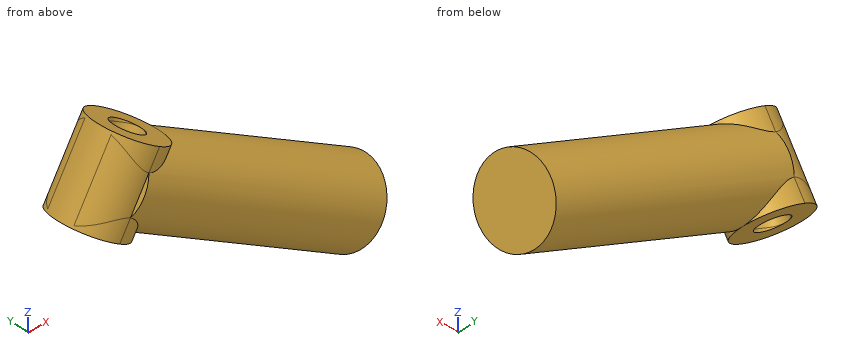
```python
from build123d import *
from build123d.topology import SkipClean

# Parameters (mm, degrees)
BOSS_EXTRUDE1_DEPTH = 25
SKETCH2_R           = 8
CUT_EXTRUDE1_DEPTH  = 110
CUT_EXTRUDE2_DEPTH  = 150
BOSS_EXTRUDE2_START = 21.60254038
BOSS_EXTRUDE2_DEPTH = 21.60254038
SKETCH5_R           = 13
CUT_EXTRUDE3_DEPTH  = 50
SKETCH6_R           = 13
BOSS_EXTRUDE3_DEPTH = 100
SKETCH7_R           = 5
CUT_EXTRUDE4_DEPTH  = 50
SKETCH8_R           = 11.5
SKETCH8_R_2         = 5
BOSS_EXTRUDE4_DEPTH = 13
CUT_EXTRUDE5_DEPTH  = 28


with BuildPart() as part:
    # Sketch1 → Boss-Extrude1 (new, symmetric)
    with BuildSketch(Plane(origin=(0, 0, 0), x_dir=(1, 0, 0), z_dir=(0, 1, 0))):
        Polygon((86.602540378, 150), (103.923048454, 160), (114.724318643, 141.291651246), (93.073683549, 128.791651246), (158.073683549, 16.208348754), (179.724318643, 28.708348754), (190.525588833, 10), (173.205080757, 0), (45.59802172, 0), (22.79901086, 39.489045172), align=None)
    extrude(amount=BOSS_EXTRUDE1_DEPTH, both=True)

    # Sketch2 → Cut-Extrude1 (cut, symmetric)
    with BuildSketch(Plane(origin=(140.729128115, 0, -81.25), x_dir=(0.8660254037844386, 0, -0.5000000000000003), z_dir=(0.5000000000000003, 0, 0.8660254037844386))):
        Circle(SKETCH2_R)
    extrude(amount=CUT_EXTRUDE1_DEPTH, both=True, mode=Mode.SUBTRACT)

    # Sketch3 → Cut-Extrude2 (cut, symmetric)
    with BuildSketch(Plane(origin=(140.729128115, 0, -81.25), x_dir=(0.8660254037844386, 0, -0.5000000000000003), z_dir=(0.5000000000000003, 0, 0.8660254037844386))):
        with BuildLine():
            Line((0, 18), (-12.5, 18))
            Line((-12.5, 18), (-12.5, 31.312178452))
            Line((-12.5, 31.312178452), (23.905899442, 31.312178452))
            Line((23.905899442, 31.312178452), (23.905899442, -29.505210198))
            Line((23.905899442, -29.505210198), (-12.5, -29.505210198))
            Line((-12.5, -29.505210198), (-12.5, -18))
            Line((-12.5, -18), (0, -18))
            ThreePointArc((0, -18), (18, 0), (0, 18))
        make_face()
    extrude(amount=CUT_EXTRUDE2_DEPTH, both=True, mode=Mode.SUBTRACT)

    # Sketch4 → Boss-Extrude2 (add)
    with SkipClean():  # the faces are left unmerged after this step: merging them gives an invalid solid
        with BuildSketch(Plane(origin=(173.229128115, 0, -24.958348754), x_dir=(0.8660254037844386, 0, -0.5000000000000003), z_dir=(0.5000000000000003, 0, 0.8660254037844386)).offset(BOSS_EXTRUDE2_START)):
            with BuildLine():
                Line((7.5, 16.363068172), (7.5, 2.783882181))
                ThreePointArc((7.5, 2.783882181), (8, 0), (7.5, -2.783882181))
                Line((7.5, -2.783882181), (7.5, -16.363068172))
                ThreePointArc((7.5, -16.363068172), (18, 0), (7.5, 16.363068172))
            make_face()
        boss_extrude2 = extrude(amount=-BOSS_EXTRUDE2_DEPTH)

    # Mirror2: Boss-Extrude2 across plane
    with SkipClean():  # the faces are left unmerged after this step: merging them gives an invalid solid
        add(boss_extrude2.mirror(Plane(origin=(140.729128115, 0, -81.25), x_dir=(-0.8660254037844388, 0, 0.5), z_dir=(0.5000000000000003, 0, 0.8660254037844386))))

    # Sketch5 → Cut-Extrude3 (cut)
    with SkipClean():  # the faces are left unmerged after this step: merging them gives an invalid solid
        with BuildSketch(Plane(origin=(34.19851629, 0, -19.744522586), x_dir=(0.5000000000000001, 0, 0.8660254037844386), z_dir=(-0.8660254037844386, 0, 0.5000000000000001))):
            Circle(SKETCH5_R)
        extrude(amount=-CUT_EXTRUDE3_DEPTH, mode=Mode.SUBTRACT)


with BuildPart() as body_2:
    # Sketch6 → Boss-Extrude3 (new body)
    with BuildSketch(Plane(origin=(77.499786479, 0, -44.744522586), x_dir=(0.5000000000000001, 0, 0.8660254037844386), z_dir=(-0.8660254037844386, 0, 0.5000000000000001))):
        with Locations(Location((0, 0, 0), (0, 0, 180))):
            Circle(SKETCH6_R)
    extrude(amount=BOSS_EXTRUDE3_DEPTH)

    # Sketch7 → Cut-Extrude4 (cut, symmetric)
    with BuildSketch(Plane(origin=(140.729128115, 0, -81.25), x_dir=(0.8660254037844386, 0, -0.5000000000000003), z_dir=(0.5000000000000003, 0, 0.8660254037844386))):
        with Locations(Location((-162.5, 0, 0), (0, 0, 180.000000003))):
            Circle(SKETCH7_R)
    extrude(amount=CUT_EXTRUDE4_DEPTH, both=True, mode=Mode.SUBTRACT)

    # Sketch8 → Boss-Extrude4 (add, symmetric)
    with BuildSketch(Plane(origin=(140.729128115, 0, -81.25), x_dir=(0.8660254037844386, 0, -0.5000000000000003), z_dir=(0.5000000000000003, 0, 0.8660254037844386))):
        with Locations((-162.5, 0)):
            Circle(SKETCH8_R)
        with Locations((-162.5, 0)):
            Circle(SKETCH8_R_2, mode=Mode.SUBTRACT)
    extrude(amount=BOSS_EXTRUDE4_DEPTH, both=True)

    # Sketch9 → Cut-Extrude5 (cut, symmetric)
    with BuildSketch(Plane(origin=(140.729128115, 0, -81.25), x_dir=(0.8660254037844386, 0, -0.5000000000000003), z_dir=(0.5000000000000003, 0, 0.8660254037844386))):
        with BuildLine():
            Line((-162.5, 11.5), (-162.5, 18.834095503))
            ThreePointArc((-162.5, 18.834095503), (-181.334095503, 0), (-162.5, -18.834095503))
            Line((-162.5, -18.834095503), (-162.5, -11.5))
            ThreePointArc((-162.5, -11.5), (-174, 0), (-162.5, 11.5))
        make_face()
    extrude(amount=CUT_EXTRUDE5_DEPTH, both=True, mode=Mode.SUBTRACT)


solid = body_2.part
```
Source: CAD feature listing. Evaluate the final solid. Frame: model axes, mm. Coordinates: 2 decimals unless noted, no trailing zeros. Write each loop counter-clockwise with the first axis right and the second up, starting at its lowest first coordinate (ties: lowest second). Pieces come first, ordered by that corner, then holes. Notation, with made-up numbers: (76.25, 72.25) -> (121.25, 72.25) arc R15 ccw to (121.25, 100.25) -> close; hole circle Ø1 at (47.5, 2.25). An arc over 180 degrees is marked (long way). Return JSON: item names as keys, results as strings. Group by question number.
1) Contact query for flat-ended pins moving along their axis: P1, Ø1, axis at x = 23.5, y = -2, coming from the +Z side; P2, Ø2, axis at x = 23.5, y = 7.5, coming from the +Z side; P3, Ø5, axis at x = 72.5, y = 6.5, coming from the +Z side. Output: stop coordinate, or through.
2) Ray query, line 1 along X through (y, z) = (-0.5, 13.5); line 2 along Y through (x, z) = (4.5, 3.5); line 3 along X through (y, z) = (2.25, -1.5). Return the intervals inside material, ascending.
3) Section query A-A, the plane y = -2.5. Return loops of the section in (x, z), plus the area to 3 significant figures.
4) Section query B-B, the plane y = 9.25. Return loops of the section in (x, z).
From the geometry:
{
 "1": {"P1": "z = 1.57", "P2": "z = -0.36", "P3": "z = -26.84"},
 "2": {"line 1": "-5.47 to 2.05", "line 2": "-11.88 to -4.52, 4.52 to 11.88", "line 3": "-13.89 to -6.02, 4.29 to 28.21"},
 "3": {"outline": "(-16.22, -5.65) -> (-10.25, -9.09) -> (2.75, 13.42) -> (-3.22, 16.87) -> close; (-2.75, -13.42) -> (3.22, -16.87) -> (3.34, -16.66) -> (71.12, -55.79) -> (83.88, -33.7) -> (16.1, 5.44) -> (16.22, 5.65) -> (10.25, 9.09) -> close", "area": "2,360 mm²"},
 "4": {"outline": "(-12.42, -7.84) -> (-0.58, -14.67) -> (1.35, -11.33) -> (72.93, -52.66) -> (82.07, -36.83) -> (10.48, 4.49) -> (12.42, 7.84) -> (0.58, 14.67) -> close"}
}
